For this review, take the finished solid that the model builds, in its own axes (mm). Give positions to 0.01 mm unless a question says otherwise; leave off trailing zeros. Write each loop counter-clockwise with the first axis right and the second up, starting at its lowest first coordinate (ties: lowest second). Pieces come first, ordered by that corner, then holes.
Q1. We need section D-D (x = -312.5). Write out the cut boundary in (y, z) (3 decimals), then the cut area to 3 significant figures.
Q2. Mouldability with a two-part tool opening along Y and no side actions: class faces 1 (the cylindrical face through (-362.746, 0.41, 1.565)), 2 (the cylindrical face through (15.57, 12.98, 1.57)), 3 (the flat face through (-15.962, -27.105, 1.565)), 4 (the cylindrical face through (-324.953, -10.594, 1.565)) as released by +Y, released by -Y, zero draft, split by the parting line, or undercut.
Q3. Insertion check: P1, Ø1, axis at y = -20, z = 2, coming from the -X side; P2, Ø3, axis at x = -57.55, y = 24.61, coming from the +Z side; P3, Ø1.6, axis at x = -203.5, z = 1, coming from the -Y side. Each pin has a flat end and moves straight along its axis. Give the tip position at first contact, or say it passes through.
Q4. We need section C-C (z = 0.65). Give the number of separate pieces and of enclosed holes in the cut face, then the cut area to 3 significant figures.
Q5. We need section B-B (x = -257). Write out the cut boundary in (y, z) (3 decimals), then the cut area to 3 significant figures.
Q6. For line 1 (X direction, y = 7.5, z = 0.3); line 2 (Y direction, x = -142, z = 0.8); line 3 (X direction, y = 3.5, z = 0.6), list the stretches that pass through material, from the lowest coordinate up.
Q7. We need section A-A (x = -4.5). Write out the cut boundary in (y, z) (3 decimals).
```python
from build123d import *

# Parameters (mm, degrees)
F0_R     = 1.7272
F0_R_2   = 3.96875
F0_R_3   = 11.1125
F1_DEPTH = 3.175
F3_DEPTH = 3.175
F4_COUNT = 6
F4_ANGLE = 300


with BuildPart() as f1:
    # F0 (on Top) → F1 (new body)
    with BuildSketch(Plane.XY):
        with BuildLine():
            Line((-303.6125627, 32.54375), (-346.1094200534, 21.5120031198))
            ThreePointArc((-346.1094200534, 21.5120031198), (-362.7501254, 0), (-346.1094200534, -21.5120031198))
            Line((-346.1094200534, -21.5120031198), (-303.6125627, -32.54375))
            Line((-303.6125627, -32.54375), (-297.2625627, -32.54375))
            Line((-297.2625627, -32.54375), (-297.2625627, -29.36875))
            Line((-297.2625627, -29.36875), (-43.2625627, -29.36875))
            Line((-43.2625627, -29.36875), (-43.2625627, -32.54375))
            Line((-43.2625627, -32.54375), (-36.9125627, -32.54375))
            Line((-36.9125627, -32.54375), (5.5842946534, -21.5120031198))
            ThreePointArc((5.5842946534, -21.5120031198), (22.225, 0), (5.5842946534, 21.5120031198))
            Line((5.5842946534, 21.5120031198), (-36.9125627, 32.54375))
            Line((-36.9125627, 32.54375), (-43.2625627, 32.54375))
            Line((-43.2625627, 32.54375), (-43.2625627, 29.36875))
            Line((-43.2625627, 29.36875), (-297.2625627, 29.36875))
            Line((-297.2625627, 29.36875), (-297.2625627, 32.54375))
            Line((-297.2625627, 32.54375), (-303.6125627, 32.54375))
        make_face()
        with Locations((-282.9750627, -24.60625)):
            Circle(F0_R, mode=Mode.SUBTRACT)
        with Locations((-352.3117115589, -11.7865861589)):
            Circle(F0_R, mode=Mode.SUBTRACT)
        with Locations((-328.7385392411, -11.7865861589)):
            Circle(F0_R_2, mode=Mode.SUBTRACT)
        with Locations((-57.5500627, -24.60625)):
            Circle(F0_R, mode=Mode.SUBTRACT)
        with Locations((-11.7865861589, -11.7865861589)):
            Circle(F0_R_2, mode=Mode.SUBTRACT)
        with Locations((11.7865861589, -11.7865861589)):
            Circle(F0_R, mode=Mode.SUBTRACT)
        with Locations((-340.5251254, 0)):
            Circle(F0_R_3, mode=Mode.SUBTRACT)
        with Locations((-289.7251254, 0)):
            Circle(F0_R, mode=Mode.SUBTRACT)
        with Locations((-352.3117115589, 11.7865861589)):
            Circle(F0_R_2, mode=Mode.SUBTRACT)
        with Locations((-328.7385392411, 11.7865861589)):
            Circle(F0_R, mode=Mode.SUBTRACT)
        with Locations((-282.9750627, 24.60625)):
            Circle(F0_R, mode=Mode.SUBTRACT)
        with Locations((-50.8, 0)):
            Circle(F0_R, mode=Mode.SUBTRACT)
        Circle(F0_R_3, mode=Mode.SUBTRACT)
        with Locations((-11.7865861589, 11.7865861589)):
            Circle(F0_R, mode=Mode.SUBTRACT)
        with Locations((11.7865861589, 11.7865861589)):
            Circle(F0_R_2, mode=Mode.SUBTRACT)
        with Locations((-57.5500627, 24.60625)):
            Circle(F0_R, mode=Mode.SUBTRACT)
    extrude(amount=F1_DEPTH)

    # F2 (on face) → F3 (cut, through all)
    with BuildSketch(Plane(origin=(0, 0, 0), x_dir=(1, 0, 0), z_dir=(0, 0, -1))):
        with BuildLine():
            ThreePointArc((-348.3828495059, -7.8577241059), (-350.1488326996, -5.55625), (-351.2589761446, -2.8761266387))
            Line((-351.2589761446, -2.8761266387), (-352.0256797693, -3.0815642558))
            ThreePointArc((-352.0256797693, -3.0815642558), (-350.8362403638, -5.953125), (-348.9441155135, -8.4189901135))
            Line((-348.9441155135, -8.4189901135), (-348.3828495059, -7.8577241059))
        make_face()
    f3 = extrude(amount=-F3_DEPTH, mode=Mode.SUBTRACT)

    # F4: F3 ×6 about axis
    f4_axis = Axis((-340.5251254, 0, 0), (0, 0, -1))
    for i in range(1, F4_COUNT):
        add(f3.rotate(f4_axis, i * F4_ANGLE / (F4_COUNT - 1)), mode=Mode.SUBTRACT)


solid = f1.part
```
Computed:
1. outline: (-30.237, 0) - (30.237, 0) - (30.237, 3.175) - (-30.237, 3.175) - close
1. area: 192 mm2
2. face 1: split by the parting line
2. face 2: undercut
2. face 3: released by -Y
2. face 4: undercut
3. P1: stops at x = -351.19
3. P2: passes through
3. P3: stops at y = -29.37
4. separate pieces: 1
4. enclosed holes: 16
4. area: 20,300 mm2
5. outline: (-29.369, 0) - (29.369, 0) - (29.369, 3.175) - (-29.369, 3.175) - close
5. area: 186 mm2
6. line 1: x = -361.45 to -349.77, -331.28 to -8.2, 8.2 to 20.92
6. line 2: y = -29.37 to 29.37
6. line 3: x = -362.47 to -351.91, -329.14 to -10.55, 10.55 to 21.95
7. outline: (-24.13, 0) - (-10.161, 0) - (-10.161, 3.175) - (-24.13, 3.175) - close; (10.161, 0) - (24.13, 0) - (24.13, 3.175) - (10.161, 3.175) - close
